from build123d import *

# Parameters (mm, degrees)
SKETCH1_R                            = 4
BOSS_EXTRUDE1_DEPTH                  = 80
SKETCH2_W                            = 5.405623026
SKETCH2_H                            = 2.438582992
BOSS_EXTRUDE3_DEPTH                  = 2.5
BOSS_EXTRUDE3_DIRECTION_2_REACH      = 82.498
BOSS_EXTRUDE3_DIRECTION_2_END_RADIUS = 4
FILLET2_R                            = 0.2


with BuildPart() as part:
    # Sketch1 → Boss-Extrude1 (new body)
    with BuildSketch(Plane(origin=(0, 0, 0), x_dir=(0, 0, -1), z_dir=(1, 0, 0))):
        Circle(SKETCH1_R)
    extrude(amount=BOSS_EXTRUDE1_DEPTH)

    # Sketch2 → Boss-Extrude3 (add)
    with BuildSketch(Plane(origin=(0, 4, 0), x_dir=(1, 0, 0), z_dir=(0, 1, 0))):
        with Locations((60.729644263, 0)):
            Rectangle(SKETCH2_W, SKETCH2_H)
    extrude(amount=BOSS_EXTRUDE3_DEPTH)

    # Boss-Extrude3 direction 2: up to this cylinder (the profile starts outside it)
    boss_extrude3_direction_2_end = Plane(origin=(60.729644, 0, 0), z_dir=(-1, 0, 0)) * Cylinder(BOSS_EXTRUDE3_DIRECTION_2_END_RADIUS, 173.996, mode=Mode.PRIVATE)
    # Sketch2 → Boss-Extrude3 direction 2 (add, up to the surface)
    with BuildSketch(Plane(origin=(0, 4, 0), x_dir=(1, 0, 0), z_dir=(0, 1, 0)), mode=Mode.PRIVATE) as boss_extrude3_direction_2_sk1:
        with Locations((60.729644263, 0)):
            Rectangle(SKETCH2_W, SKETCH2_H)
    boss_extrude3_direction_2_tool1 = extrude(boss_extrude3_direction_2_sk1.sketch, amount=-BOSS_EXTRUDE3_DIRECTION_2_REACH, mode=Mode.PRIVATE) - boss_extrude3_direction_2_end
    add(boss_extrude3_direction_2_tool1.solids().sort_by_distance((60.729644, 4, 0))[0])
    add(boss_extrude3_direction_2_tool1.solids().sort_by_distance((60.729644, 4, 0))[1])

    # Fillet2
    fillet2_edges = [part.edges().sort_by_distance(p)[0] for p in [
        (63.432455776, 6.5, 0),
        (58.02683275, 6.5, 0),
    ]]
    fillet(fillet2_edges, radius=FILLET2_R)


solid = part.part
Geometry: final body of the model. Coordinates: model frame, mm. A direction names the side the tool comes from. Give positions to 0.01 mm unless a question says otherwise; leave off trailing zeros. Write each loop counter-clockwise with the first axis right and the second up, starting at its lowest first coordinate (ties: lowest second). Pieces come first, ordered by that corner, then holes. Notation, with made-up numbers: (51.5, 10) - (61.5, 10) arc R5 cw to (61.5, 15) - close; hole circle Ø2 at (47.25, 85.5). An arc over 180 degrees is marked (long way). Return JSON: item names as keys, results as strings. Group by question number.
1) First-contact query: P1, Ø3, axis at x = 60, y = 5.5, coming from the +Z side; P2, Ø2, axis at x = 8.5, z = -1, coming from the -Y side; P3, Ø0.7, axis at y = 4.5, z = -0.5, coming from the +X side; P4, Ø3, axis at x = 36.5, y = 2.5, coming from the -Z side. Flat tips, straight axial feed; report the tip coordinate or a pass-through.
2) Section A-A on z = 0. Return the cut outline in (x, y).
3) Section C-C on y = -2.75. Return the cut outline in (x, z).
4) Line query: line 1 (Y direction, x = 37, z = 0.25); line 2 (Y direction, x = 29, z = 1); line 3 (Z direction, x = 73.5, y = 1.5). Output: solid intervals per line, ascending.
5) Set-up query: faces 1 (the flat face through (61, 5, 1.219)), 2 (the flat face through (61, 6.5, 0)), 3 (the flat face through (61, 5, -1.219)). Return all of +Z, -Z, +X, -X, +Y, -Y with unobstructed straight access to the full face (end or side cutting, diameter ignored); none if empty.
6) Section B-B on x = 44. Return the cut outline in (y, z), plus the area to 3 significant figures.
Filled in:
{
 "1": {"P1": "stops at z = 1.22", "P2": "stops at y = -4", "P3": "stops at x = 63.43", "P4": "stops at z = -3.87"},
 "2": {"outline": "(0, -4) - (80, -4) - (80, 4) - (63.43, 4) - (63.43, 6.3) arc R0.2 ccw to (63.23, 6.5) - (58.23, 6.5) arc R0.2 ccw to (58.03, 6.3) - (58.03, 4) - (0, 4) - close"},
 "3": {"outline": "(0, -2.9) - (80, -2.9) - (80, 2.9) - (0, 2.9) - close"},
 "4": {"line 1": "y = -3.99 to 3.99", "line 2": "y = -3.87 to 3.87", "line 3": "z = -3.71 to 3.71"},
 "5": {"face 1": "+Z, +X, -X, +Y", "face 2": "+Z, -Z, +X, -X, +Y", "face 3": "-Z, +X, -X, +Y"},
 "6": {"outline": "circle Ø8 at (0, 0)", "area": "50.3 mm^2"}
}
